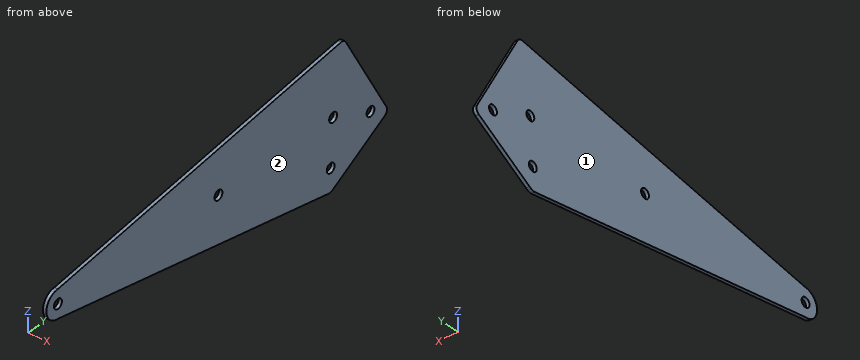
Autodesk Inventor part; units mm, degrees
ref_plane "YZ Plane" through (0, 0, 0) normal (1, 0, 0) x (0, 1, 0)
ref_plane "XZ Plane" through (0, 0, 0) normal (0, 1, 0) x (-1, 0, 0)
ref_plane "XY Plane" through (0, 0, 0) normal (0, 0, 1) x (1, 0, 0)
sketch "Sketch1" plane through (0, 0, 0) normal (1, 0, 0) x (0, 1, 0)
  circle A0 centre (-86.8757, 0.9387) radius 2.1844
  circle A1 centre (2.0243, 0.9387) radius 2.1844
  circle A2 centre (65.5243, 0.9387) radius 2.1844
  circle A3 centre (64.1826, -19.9575) radius 2.1844
  circle A4 centre (86.2299, -7.3449) radius 2.1844
  line L0 (65.9484, -29.438) -> (95.1218, -12.7487)
  circle A5 centre (64.1826, -19.9575) radius 2.1844
  circle A6 centre (65.5243, 0.9387) radius 2.1844
  circle A7 centre (86.2299, -7.3449) radius 2.1844
  circle A8 centre (2.0243, 0.9387) radius 2.1844
  circle A9 centre (-86.8757, 0.9387) radius 2.1844
  circle A10 centre (-86.8757, 0.9387) radius 6.35
  line L1 (-86.8757, -5.4113) -> (63.0678, -30.2634)
  line L2 (65.1635, -29.887) -> (94.0863, -13.341)
  line L3 (95.0298, -9.8751) -> (72.5412, 29.4356)
  line L4 (69.9617, 30.6865) -> (-86.8757, 7.2887)
  arc A11 (63.0678, -30.2634) -> (65.1635, -29.887) centre (63.5869, -27.1311) ccw
  arc A12 (94.0863, -13.341) -> (95.0298, -9.8751) centre (92.8251, -11.1363) ccw
  arc A13 (72.5412, 29.4356) -> (69.9617, 30.6865) centre (70.3364, 28.1743) ccw
  point P0 (0, 0)
  point P1 (96.291, -12.0798)
  dimension "d0" = 12.7
  dimension "d1" = 3.175
  dimension "d2" = 2.54
extrude "Extrusion1" add sketch "Sketch1" along normal blind 1.5875
properties part number "prerollernew"
Model file for the job. Use its own axes, mm. Face numbers are marked on the shaded views. Give positions to 0.01 mm unless a question says otherwise; leave off trailing zeros. Loops run counter-clockwise (first coordinate to the right, second up) from the corner with the lowest first, then second, coordinate; pieces in that order, holes last. Notation, with made-up numbers: (76, 22.5) -> (135, 22.5) arc R19 cw to (135, 46.5) -> close; hole circle Ø4 at (-27.75, 47.5). An arc over 180 degrees is marked (long way). Use a Markdown table: item, result. Add a question column.
(1) Slice it at B-B on y = 55. List the corners of the cut face in (x, z).
(2) Mould opens along X. For the marked faces 1 and 2 say: +X half, -X half, draft (parallel to the pull), parting line (faces both ways), or undercut.
(3) Slice it at C-C on z = -3.5. List the corners of the cut face in (x, y).
(4) Wall check: line 1 along Z through (x, y) = (1.4, 65); line 2 along Z through (x, y) = (1.15, -68.5); line 3 along Z through (x, y) = (0.9, -74.5). Give the ranges that are in metal, low to high.
(5) Slice it at A-A on x = 1.3. List the corners of the cut face in (y, z).
(6) Drop a flat-ended pin along its axis: pin 1 Ø5 at (y, z) = (2.02, 0.94) entering from -X. Give the stop position or say it passes through.
Filled sheet:
| question | item | result |
|---|---|---|
| 1 | outline | (0, -28.93) -> (1.59, -28.93) -> (1.59, 28.45) -> (0, 28.45) -> close |
| 2 | face 1 | -X half |
| 2 | face 2 | +X half |
| 3 | outline | (0, -91.42) -> (1.59, -91.42) -> (1.59, 91.38) -> (0, 91.38) -> close |
| 4 | line 1 | -29.97 to -21.98, -17.93 to -1.18, 3.06 to 29.95 |
| 4 | line 2 | -8.46 to 10.03 |
| 4 | line 3 | -7.46 to 9.13 |
| 5 | outline | (-86.88, -5.41) -> (63.07, -30.26) arc R3.17 ccw to (65.16, -29.89) -> (65.95, -29.44) -> (94.09, -13.34) arc R2.54 ccw to (95.03, -9.88) -> (72.54, 29.44) arc R2.54 ccw to (69.96, 30.69) -> (-86.88, 7.29) arc R6.35 ccw to start; hole circle Ø4.37 at (-86.88, 0.94); hole circle Ø4.37 at (2.02, 0.94); hole circle Ø4.37 at (64.18, -19.96); hole circle Ø4.37 at (65.52, 0.94); hole circle Ø4.37 at (86.23, -7.34) |
| 6 | pin 1 | x = 0 |
